```python
from build123d import *

# Parameters (mm, degrees)
SALIENTE_EXTRUIR1_DEPTH = 15
CROQUIS3_R              = 14.29
CORTAR_EXTRUIR2_DEPTH   = 499.221807184


with BuildPart() as part:
    # Croquis1 → Saliente-Extruir1 (new body)
    with BuildSketch(Plane(origin=(0, 0, 0), x_dir=(1, 0, 0), z_dir=(0, 1, 0))):
        with BuildLine():
            Line((28.62028588, 380.086840422), (-203.253807163, -15.179678662))
            ThreePointArc((-203.253807163, -15.179678662), (-244.309678662, -25.876192837), (-255.006192837, 15.179678662))
            Line((-255.006192837, 15.179678662), (-23.132099794, 410.446197745))
            ThreePointArc((-23.132099794, 410.446197745), (17.923771705, 421.142711921), (28.62028588, 380.086840422))
        make_face()
    extrude(amount=SALIENTE_EXTRUIR1_DEPTH)

    # Croquis3 → Cortar-Extruir2 (cut, through all)
    with BuildSketch(Plane(origin=(0, 15, 0), x_dir=(1, 0, 0), z_dir=(0, 1, 0))):
        with Locations(Location((-229.13, 0, 0), (0, 0, 270))):
            Circle(CROQUIS3_R)
        with Locations(Location((2.744093043, 395.266519084, 0), (0, 0, 270))):
            Circle(CROQUIS3_R)
    extrude(amount=-CORTAR_EXTRUIR2_DEPTH, mode=Mode.SUBTRACT)


solid = part.part
```
The model under review builds one solid part; all positions refer to its coordinate system, in mm. Round coordinates to 2 decimals unless told otherwise and drop trailing zeros. Order: outer loops, then holes, each group sorted by start corner. A loop starts at its lowest first (then second) coordinate and runs counter-clockwise, first axis right, second up. Notation, with made-up numbers: M 24.5,-37.75 L 66.5,-37.75 A26 cw 66.5,-9.75 Z; hole C 86,34 d6. An arc over 180 degrees is marked long. Use a Markdown table: item, result.
1) Consider section C-C (y = 4.5). Write out the cut boundary in (x, z).
Report:
| item | result |
|---|---|
| outline | M -255.01,-15.18 L -23.13,-410.45 A30 ccw 28.62,-380.09 L -203.25,15.18 A30 ccw Z; hole C -229.13,0 d28.58; hole C 2.74,-395.27 d28.58 |
2) Consider section A-A (x = -229.13). Write out the cut boundary in (y, z).
Report:
| item | result |
|---|---|
| outline | M 0,-59.29 L 15,-59.29 L 15,-14.29 L 0,-14.29 Z; M 0,14.29 L 15,14.29 L 15,30 L 0,30 Z |
3) Insertion check: pin 1 (17 mm diameter, centred on x = -229.13, z = 0, fed in from -Y); pin 2 (2 mm diameter, centred on x = -207, y = 4, fed in from +Z); pin 3 (4 mm diameter, centred on x = -103, y = 13, fed in from +Z); pin 4 (6 mm diameter, centred on y = 13, z = -75, fed in from +X). Each pin has a flat end and moves straight along its axis. Give the tip position at first contact, or say it passes through.
Report:
| item | result |
|---|---|
| pin 1 | through |
| pin 2 | z = 21.3 |
| pin 3 | z = -152.31 |
| pin 4 | x = -148.59 |
4) Draft analysis for pull direction Z (two halves, no side actions). For faces 1 (the face through (3.372, 7.605, -409.543)), 2 (the face through (-113, 0, -199)), 3 (the face through (-214.96, 7.6, -1.86)), 4 (the face through (-140.69, 7.4, -210.05)), state which applies: released by +Z, released by -Z, zero draft, split by the parting line, or undercut.
Report:
| item | result |
|---|---|
| face 1 | undercut |
| face 2 | zero draft |
| face 3 | undercut |
| face 4 | released by -Z |
5) Wall thickness on line 1 along X through (y, z) = (12.5, -404.5); line 2 along Z through (x, y) = (5, 11); line 3 along Z through (x, y) = (-29.5, 12.25): over which ranges is each line inside the solid? List them lowest first. Write a range as [from, to].
Report:
| item | result |
|---|---|
| line 1 | [-26.62, -8.16], [13.65, 31.29] |
| line 2 | [-425.18, -409.38], [-381.16, -339.82] |
| line 3 | [-399.59, -281.01] |
6) Consider section D-D (z = -94.5). Write out the cut boundary in (x, y), then the cut area to 3 significant figures.
Report:
| item | result |
|---|---|
| outline | M -208.47,0 L -138.91,0 L -138.91,15 L -208.47,15 Z |
| area | 1,040 mm^2 |
7) Consider section B-B (z = 0). Write out the cut boundary in (x, y).
Report:
| item | result |
|---|---|
| outline | M -259.13,0 L -243.42,0 L -243.42,15 L -259.13,15 Z; M -214.84,0 L -194.35,0 L -194.35,15 L -214.84,15 Z |
